Study the drawing (mm; zero at the part's minimum x, y, z) and answer. Give positions to 0.01 mm unless a question says otherwise; leave off trailing zeros. Write each loop counter-clockwise with the first axis right and the second up, starting at its lowest first coordinate (ties: lowest second). Pieces come first, ordered by that corner, then holes. Notation, with made-up numbers: (27, 6) - (36, 6) arc R16 cw to (36, 32) - close; hole circle Ø2 at (-36.5, -5). An arc over 180 degrees is marked (long way). Write each question's results on one line, items separated by ' | '. Start each with the question number.
Q1. Section D-D (x = 19.5) is taken. Determine the outline of the cut face in (y, z), plus the area to 3 significant figures.
Q2. A flat-ended cylindrical pin translates along its axis: pin 1 Ø5 at (x, z) = (56, 4.5) entering from +Y. Find the tip coordinate at first contact, or state that the pin passes through.
Q3. Section C-C (z = 2.75) is taken. State how many separate pieces and enclosed holes the cut face has, plus the area to 3 significant figures.
Q4. Section A-A (x = 115) is taken. Determine the outline of the cut face in (y, z).
Q5. Find the intervals of material crossed by probe 1 along Y at (x, z) = (20, 3.5); probe 2 along X at (y, z) = (180, 7.5); probe 3 along X at (y, z) = (20, 3.5), in increasing order.
Q6. Section B-B (y = 20) is taken. Determine the outline of the cut face in (x, z).
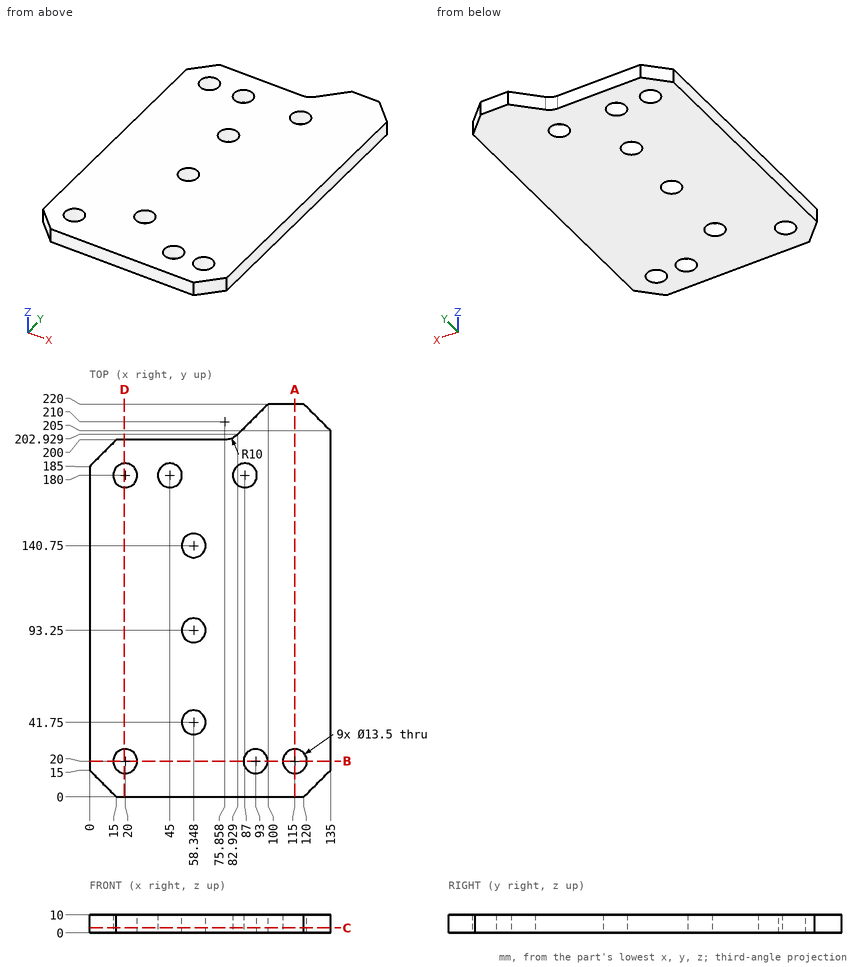
Answers below:
1) outline: (0, 0) - (13.27, 0) - (13.27, 10) - (0, 10) - close; (26.73, 0) - (173.27, 0) - (173.27, 10) - (26.73, 10) - close; (186.73, 0) - (200, 0) - (200, 10) - (186.73, 10) - close | area: 1,730 mm2
2) pin 1: stops at y = 200
3) separate pieces: 1 | enclosed holes: 9 | area: 26,200 mm2
4) outline: (0, 0) - (13.25, 0) - (13.25, 10) - (0, 10) - close; (26.75, 0) - (220, 0) - (220, 10) - (26.75, 10) - close
5) probe 1: y = 0 to 13.25, 26.75 to 173.25, 186.75 to 200 | probe 2: x = 0 to 13.25, 26.75 to 38.25, 51.75 to 80.25, 93.75 to 135 | probe 3: x = 0 to 13.25, 26.75 to 86.25, 99.75 to 108.25, 121.75 to 135
6) outline: (0, 0) - (13.25, 0) - (13.25, 10) - (0, 10) - close; (26.75, 0) - (86.25, 0) - (86.25, 10) - (26.75, 10) - close; (99.75, 0) - (108.25, 0) - (108.25, 10) - (99.75, 10) - close; (121.75, 0) - (135, 0) - (135, 10) - (121.75, 10) - close
